Source: three-view drawing plus pictorial views. Frame: mm from the lowest corner of the part. A direction names the side the tool comes from. Coordinates: 2 decimals unless noted, no trailing zeros. Order: outer loops, then holes, each group sorted by start corner. A loop starts at its lowest first (then second) coordinate and runs counter-clockwise, first axis right, second up. Notation, with made-up numbers: M -32.75,12.25 L -5.75,12.25 A14 cw -5.75,16.25 Z; hole C 48.5,55 d8. An arc over 180 degrees is marked long. One line per question, with ' | ' between items.
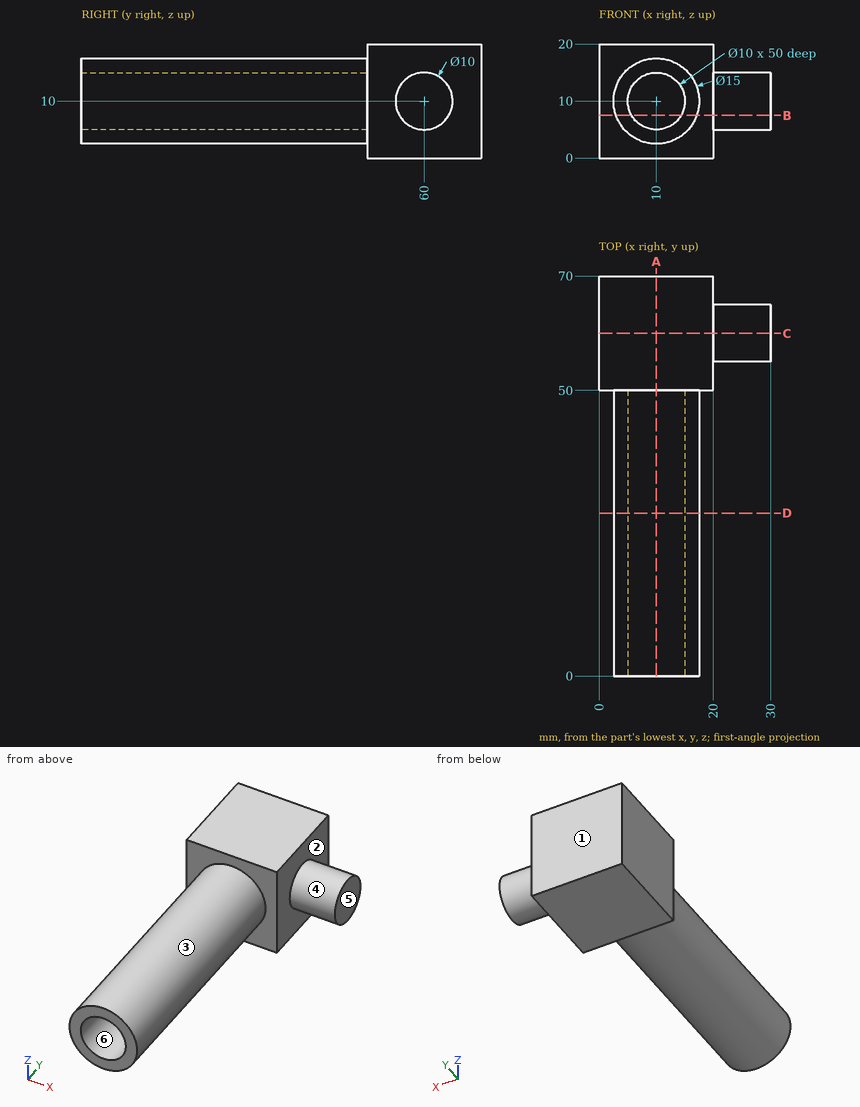
1. Pin query (flat end, axial travel): P1, Ø1.5, axis at x = 16.5, y = 33, coming from the -Z side; P2, Ø2, axis at y = 60, z = 17, coming from the +X side; P3, Ø3, axis at x = 11, z = 9.5, coming from the -Y side. Return the tip coordinate at first contact, or that it passes through.
Response values:
P1: stops at z = 5.18 | P2: stops at x = 20 | P3: stops at y = 50
2. Draft query along Z for the marked faces 4, 5 and 6. Return one class per face: pulls with the +Z half, pulls with the -Z half, needs draft (parallel to the pull), parting line crosses it, or undercut.
Response values:
face 4: parting line crosses it | face 5: needs draft | face 6: undercut
3. Section B-B, the plane z = 7.5. Output: boundary loops of the cut face in (x, y).
Response values:
outline: M 0,50 L 2.93,50 L 2.93,0 L 5.67,0 L 5.67,50 L 14.33,50 L 14.33,0 L 17.07,0 L 17.07,50 L 20,50 L 20,55.67 L 30,55.67 L 30,64.33 L 20,64.33 L 20,70 L 0,70 Z
4. Section D-D, the plane y = 28.5. Output: boundary loops of the cut face in (x, z).
Response values:
outline: C 10,10 d15; hole C 10,10 d10
5. Section A-A, the plane x = 10. Output: boundary loops of the cut face in (y, z), and give its area (3 significant figures).
Response values:
outline: M 0,2.5 L 50,2.5 L 50,0 L 70,0 L 70,20 L 50,20 L 50,17.5 L 0,17.5 L 0,15 L 50,15 L 50,5 L 0,5 Z | area: 650 mm^2
6. Access query for the marked faces 1, 2 and 3. Directions: +Z, -Z, +X, -X, +Y, -Y. A direction counts if a zero-diameter tool reaches every point of the face in a straight line with its end or side. Return the directions, or none.
Response values:
face 1: +Z, -Z, +X, -X, +Y | face 2: +X | face 3: -Y
7. Material intervals for line 1 (X direction, y = 40.5, z = 10); line 2 (Y direction, x = 12, z = 11.5); line 3 (X direction, y = 41, z = 6), sorted ascending. Write a range as [from, to].
Response values:
line 1: x = [2.5, 5], [15, 17.5] | line 2: y = [50, 70] | line 3: x = [3.66, 7], [13, 16.34]
8. Section C-C, the plane y = 60. Output: boundary loops of the cut face in (x, z), and give its area (3 significant figures).
Response values:
outline: M 0,0 L 20,0 L 20,5 L 30,5 L 30,15 L 20,15 L 20,20 L 0,20 Z | area: 500 mm^2
